from build123d import *

# Parameters (mm, degrees)
STOCK_OUTTER_CASE_1_START = -4
STOCK_OUTTER_CASE_1_DEPTH = 184.8
FILLET1_R                 = 0.2
BOSS_EXTRUDE4_DEPTH       = 29.8
FILLET3_R                 = 0.3
FILLET4_R                 = 1


# Read off the part's stored shape, not the designer's step: Stock-outter_case-1
with BuildPart() as part:
    # Stock-outter_case-1 outline → Stock-outter_case-1 (new body)
    with BuildSketch(Plane(origin=(0, 0, 0), x_dir=(1, 0, 0), z_dir=(0, 1, 0)).offset(STOCK_OUTTER_CASE_1_START)):
        with BuildLine():
            Line((-138, 93), (-135, 93))
            Line((-135, 93), (-135, 96))
            Line((-135, 96), (-138, 96))
            ThreePointArc((-138, 96), (-150.727922061, 90.727922061), (-156, 78))
            Line((-156, 78), (-156, 75))
            Line((-156, 75), (-153, 75))
            Line((-153, 75), (-153, 78))
            ThreePointArc((-153, 78), (-148.606601718, 88.606601718), (-138, 93))
        make_face()
    extrude(amount=STOCK_OUTTER_CASE_1_DEPTH)

    # Fillet1
    fillet1_edges = [part.edges().sort_by_distance(p)[0] for p in [
        (-150.727922061, 180.8, -90.727922061),
        (-156, 180.8, -76.5),
        (-136.5, 180.8, -96),
        (-150.727922061, -4, -90.727922061),
        (-156, -4, -76.5),
        (-136.5, -4, -96),
        (-156, 88.4, -75),
        (-135, 88.4, -96),
    ]]
    fillet(fillet1_edges, radius=FILLET1_R)

    # Sketch5 → Boss-Extrude4 (add, symmetric)
    with BuildSketch(Plane(origin=(0, 74, 0), x_dir=(1, 0, 0), z_dir=(0, 1, 0))):
        with BuildLine():
            Line((-137.385981926, 79.358072098), (-137.056795696, 81.56280876))
            ThreePointArc((-137.056795696, 81.56280876), (-137.228508787, 81.694568849), (-137.439817918, 81.741414955))
            Line((-137.439817918, 81.741414955), (-138.298334245, 81.741414955))
            ThreePointArc((-138.298334245, 81.741414955), (-139.204642032, 82.318796694), (-139.064378688, 83.384202565))
            Line((-139.064378688, 83.384202565), (-144.848487028, 91.34534471))
            ThreePointArc((-144.848487028, 91.34534471), (-146.365861195, 90.450396237), (-147.767847562, 89.383723205))
            Line((-147.767847562, 89.383723205), (-137.385981926, 79.358072098))
        make_face()
    boss_extrude4 = extrude(amount=BOSS_EXTRUDE4_DEPTH, both=True)

    # Mirror2: Boss-Extrude4 across plane
    add(boss_extrude4.mirror(Plane(origin=(-30, 0, 30), x_dir=(0.7071067811865478, 0, 0.7071067811865472), z_dir=(0.7071067811865475, 0, -0.7071067811865477))))

    # Fillet3
    fillet3_edges = [part.edges().sort_by_distance(p)[0] for p in [
        (-137.385981926, 74, -79.358072098),
        (-139.358072098, 74, -77.385981926),
    ]]
    fillet(fillet3_edges, radius=FILLET3_R)

    # Fillet4
    fillet4_edges = [part.edges().sort_by_distance(p)[0] for p in [
        (-147.767847562, 74, -89.383723205),
        (-144.848487028, 74, -91.34534471),
        (-151.34534471, 74, -84.848487028),
        (-149.383723205, 74, -87.767847562),
    ]]
    fillet(fillet4_edges, radius=FILLET4_R)


solid = part.part
Check sheet for the modelled part. Datum: model origin and axes. Units: mm. A direction names the side the tool comes from. Round coordinates to 2 decimals unless told otherwise and drop trailing zeros. Loops run counter-clockwise (first coordinate to the right, second up) from the corner with the lowest first, then second, coordinate; pieces in that order, holes last.
1. Set-up check for faces 4 (the flat face through (-143, 44.2, -86)), 5 (the flat face through (-149, 180.8, -89)), 6 (the flat face through (-149, -4, -89)), 7 (the flat face through (-146.82, 74.42, -81.56)), 8 (the flat face through (-142.513, 74.417, -84.31)): record each of +Z, -Z, +X, -X, +Y, -Y from which the full face is reachable in a straight line by a thin tool's end or side.
2. Scan lines: probe 1 along Z at (x, y) = (-137.5, 51.5); probe 2 along Y at (x, z) = (-143.25, -88.25); probe 3 along X at (y, z) = (81.5, -79.75). Record each from-to range of solid material in increasing order.
3. Mould release check, pull along X, two halves, no side actions. Record for faces 1 (the flat face through (-143, 103.8, -86)), 2 (the flat face through (-141.56, 74.42, -86.82)), 3 (the flat face through (-144.31, 74.417, -82.513)): released by +X, released by -X, zero draft, split by the parting line, or undercut.
4. Gauge pin test, flat ends, axial feed: pin 1 Ø2 at (x, z) = (-150, -81) entering from +Y; pin 2 Ø3.5 at (x, z) = (-141.5, -86.5) entering from +Y; pin 3 Ø9 at (x, z) = (-142, -83.5) entering from -Y; pin 4 Ø2.5 at (y, z) = (127.5, -76.5) entering from +X. Record the tip position at first contact, or that the pin passes through.
5. Sectioned sample at A-A on y = 163. Record the boundary of the cut face in (x, z), and give its area (3 significant figures).
Recorded:
1. face 4: +Z, +X, -Y
1. face 5: +Z, -Z, +X, -X, +Y
1. face 6: +Z, -Z, +X, -X, -Y
1. face 7: +Z, +Y, -Y
1. face 8: +Y, -Y
2. probe 1: z = -96 to -93, -81.74 to -79.69
2. probe 2: y = 44.2 to 103.8
2. probe 3: x = -155.91 to -152.9, -144.33 to -141.64, -137.79 to -137.4
3. face 1: zero draft
3. face 2: released by +X
3. face 3: undercut
4. pin 1: passes through
4. pin 2: stops at y = 103.8
4. pin 3: stops at y = 44.2
4. pin 4: stops at x = -153
5. outline: (-156, -78) arc R18 ccw to (-138, -96) - (-135.2, -96) arc R0.2 ccw to (-135, -95.8) - (-135, -93) - (-138, -93) arc R15 cw to (-153, -78) - (-153, -75) - (-155.8, -75) arc R0.2 ccw to (-156, -75.2) - close
5. area: 95.7 mm2
